from build123d import *

# Parameters (mm, degrees)
F1_DEPTH = 3
F3_DEPTH = 25
F4_W     = 3.49161
F4_H     = 1.112773
F5_DEPTH = 25
F6_R     = 2.5
F7_DEPTH = 25


with BuildPart() as f1:
    # F0 (on Front) → F1 (new body)
    with BuildSketch(Plane.XZ):
        with BuildLine():
            ThreePointArc((-34.598693, 13.199997), (-34.108076, 14.95115), (-33.942714, 16.762199))
            ThreePointArc((-33.942714, 16.762199), (-34.205836, 19.04106), (-34.981355, 21.199997))
            ThreePointArc((-34.981355, 21.199997), (-53.931293, 16.284418), (-34.598693, 13.199997))
        make_face()
        with BuildLine():
            ThreePointArc((-34.981355, 21.199997), (-34.205836, 19.04106), (-33.942714, 16.762199))
            ThreePointArc((-33.942714, 16.762199), (-34.108076, 14.95115), (-34.598693, 13.199997))
            Line((-34.598693, 13.199997), (3.018645, 13.199997))
            Line((3.018645, 13.199997), (3.018645, 21.199997))
            Line((3.018645, 21.199997), (-34.981355, 21.199997))
        make_face()
    extrude(amount=F1_DEPTH)

    # F2 (on face) → F3 (cut)
    with BuildSketch(Plane.XZ.offset(3)):
        Polygon((-30.966062, 16.508911), (-34.598693, 13.199997), (-27.952018, 13.199997), align=None)
        Polygon((-27.350497, 14.478252), (-27.952018, 13.199997), (-26.458988, 13.199997), align=None)
        Polygon((-23.940648, 14.956392), (-26.458988, 13.199997), (-22.715665, 13.199997), align=None)
        Polygon((-18.286822, 17.846175), (-22.715665, 13.199997), (-6.251452, 13.199997), (-8.381168, 17.648062), (-10.90711, 17.648062), (-12.492014, 14.733944), (-15.021867, 14.733944), align=None)
        Polygon((-6.251452, 13.199997), (2.415996, 13.199997), (1.772129, 17.432725), (-0.651208, 17.432725), (-2.190134, 15.419289), (-3.230228, 17.152779), align=None)
    extrude(amount=-F3_DEPTH, mode=Mode.SUBTRACT)

    # F4 (on face) → F5 (cut)
    with BuildSketch(Plane.XZ.offset(3)):
        with Locations((2.354657, 20.643611)):
            Rectangle(F4_W, F4_H)
    extrude(amount=-F5_DEPTH, mode=Mode.SUBTRACT)

    # F6 (on face) → F7 (cut)
    with BuildSketch(Plane.XZ.offset(3)):
        with Locations((-48.656683, 16.782803)):
            Circle(F6_R)
    extrude(amount=-F7_DEPTH, mode=Mode.SUBTRACT)


solid = f1.part
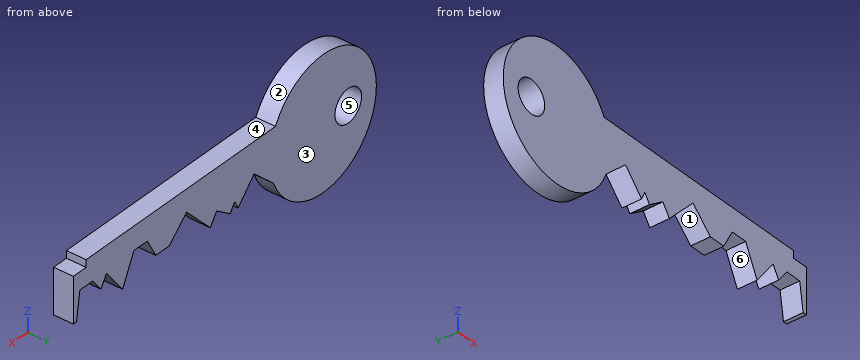
Source: CAD feature listing. Evaluate the final solid. Frame: model axes, mm. Face numbers are marked on the shaded views. A direction names the side the tool comes from. Coordinates: 2 decimals unless noted, no trailing zeros. Order: outer loops, then holes, each group sorted by start corner. A loop starts at its lowest first (then second) coordinate and runs counter-clockwise, first axis right, second up.
Item 1: Cut plane D-D (z = 11). Return loops of the section in (x, y).
Output values:
outline: (-52.12, -3) - (-35.77, -3) - (-35.77, 0) - (-52.12, 0) - close
Item 2: Pull-direction query (X, two-part tool) for the marked faces 1, 2 and 3; classes: pulls with the +X half, pulls with the -X half, needs draft (parallel to the pull), parting line crosses it, or undercut.
Output values:
face 1: undercut
face 2: parting line crosses it
face 3: needs draft
Item 3: Cut plane B-B (y = -2.3). Return loops of the section in (x, z).
Output values:
outline: (-34.98, 21.2) arc R10 ccw (long way) to (-34.6, 13.2) - (-30.97, 16.51) - (-27.95, 13.2) - (-27.35, 14.48) - (-26.46, 13.2) - (-23.94, 14.96) - (-22.72, 13.2) - (-18.29, 17.85) - (-15.02, 14.73) - (-12.49, 14.73) - (-10.91, 17.65) - (-8.38, 17.65) - (-6.25, 13.2) - (-3.23, 17.15) - (-2.19, 15.42) - (-0.65, 17.43) - (1.77, 17.43) - (2.42, 13.2) - (3.02, 13.2) - (3.02, 20.09) - (0.61, 20.09) - (0.61, 21.2) - close; hole circle Ø5 at (-48.66, 16.78)
Item 4: Cut plane A-A (x = -47.5). Return loops of the section in (y, z).
Output values:
outline: (-3, 7.42) - (0, 7.42) - (0, 14.57) - (-3, 14.57) - close; (-3, 19) - (0, 19) - (0, 26.11) - (-3, 26.11) - close
Item 5: Set-up query: the marked faces 4, 5 and 6. Return all of +Z, -Z, +X, -X, +Y, -Y with unobstructed straight access to the full face (end or side cutting, diameter ignored); none if empty.
Output values:
face 4: +Z, +X, +Y, -Y
face 5: +Y, -Y
face 6: -Z, +Y, -Y
Item 6: First-contact query: P1, Ø3, axis at x = -48.66, z = 16.78, coming from the -Y side; P2, Ø1.2, axis at x = 1, y = -1, coming from the -Z side; P3, Ø1.2, axis at x = 1.5, y = -2, coming from the +Z side. Flat tips, straight axial feed; report the tip coordinate or a pass-through.
Output values:
P1: passes through
P2: stops at z = 17.43
P3: stops at z = 20.09
Item 7: Material intervals for line 1 (X direction, y = -2.3, z = 16.75); line 2 (Z direction, x = -12.5, y = -2.75); line 3 (Z direction, x = -10, y = -2.8), sorted ascending.
Output values:
line 1: x = -53.94 to -51.16, -46.16 to -19.33, -17.14 to -11.4, -7.95 to -3.54, -2.99 to -1.17, 1.88 to 3.02
line 2: z = 14.73 to 21.2
line 3: z = 17.65 to 21.2
Item 8: Cut plane C-C (x = -28.5). Return loops of the section in (y, z).
Output values:
outline: (-3, 13.8) - (0, 13.8) - (0, 21.2) - (-3, 21.2) - close
